Source: CAD feature listing. Evaluate the final solid. Frame: model axes, mm. Face numbers are marked on the shaded views. A direction names the side the tool comes from. Coordinates: 2 decimals unless noted, no trailing zeros. Write each loop counter-clockwise with the first axis right and the second up, starting at its lowest first coordinate (ties: lowest second). Pieces come first, ordered by that corner, then holes. Notation, with made-up numbers: (51.5, -7) - (89.5, -7) arc R20 ccw to (89.5, 0) - close; hole circle Ø11 at (62, 39). An arc over 180 degrees is marked (long way). One line per item, written item: value.
from build123d import *

# Parameters (mm, degrees)
CROQUIS1_R              = 7.55
CROQUIS1_R_2            = 5
SALIENTE_EXTRUIR1_DEPTH = 7
SALIENTE_EXTRUIR2_DEPTH = 51
CROQUIS3_R              = 7.55
SALIENTE_EXTRUIR3_DEPTH = 51
CORTAR_EXTRUIR2_DEPTH   = 14.5
CROQUIS7_R              = 4.1
CORTAR_EXTRUIR3_DEPTH   = 35
CROQUIS8_W              = 8.6
CROQUIS8_H              = 23
CORTAR_EXTRUIR4_DEPTH   = 84
CROQUIS10_R             = 1.55
CORTAR_EXTRUIR7_DEPTH   = 14.5
CORTAR_EXTRUIR8_DEPTH   = 14.5
CROQUIS12_W             = 14.417096231
CROQUIS12_H             = 5
CORTAR_EXTRUIR9_DEPTH   = 14.5
CROQUIS13_W             = 9.25
CROQUIS13_H             = 13.5
SALIENTE_EXTRUIR4_DEPTH = 2.5
REDONDEO2_R             = 2
CROQUIS14_R             = 1
CORTAR_EXTRUIR10_DEPTH  = 4
CROQUIS15_R             = 1.6
CORTAR_EXTRUIR11_DEPTH  = 61.5


with BuildPart() as part:
    # Croquis1 → Saliente-Extruir1 (new body)
    with BuildSketch(Plane(origin=(0, 0, 0), x_dir=(1, 0, 0), z_dir=(0, 1, 0))):
        with BuildLine():
            Line((-11, 0), (-11, 12.5))
            Line((-11, 12.5), (-53.5, 12.5))
            Line((-53.5, 12.5), (-53.5, 26))
            Line((-53.5, 26), (29.5, 26))
            Line((29.5, 26), (29.5, 8))
            Line((29.5, 8), (29.5, 0))
            ThreePointArc((29.5, 0), (21.303512587, -11.735833137), (7.463235294, -8.0808489))
            ThreePointArc((7.463235294, -8.0808489), (-4.410465495, -10.077092543), (-11, 0))
        make_face()
        Circle(CROQUIS1_R, mode=Mode.SUBTRACT)
        with Locations((17, 0)):
            Circle(CROQUIS1_R_2, mode=Mode.SUBTRACT)
    extrude(amount=SALIENTE_EXTRUIR1_DEPTH)

    # Croquis2 → Saliente-Extruir2 (add)
    with BuildSketch(Plane.XZ):
        Polygon((29.5, -26), (29.5, -12.5), (-11, -12.5), (-53.5, -12.5), (-53.5, -26), align=None)
    extrude(amount=SALIENTE_EXTRUIR2_DEPTH)

    # Croquis3 → Saliente-Extruir3 (add)
    with BuildSketch(Plane.XZ):
        with BuildLine():
            Line((-11, 0), (-11, -12.5))
            Line((-11, -12.5), (11, -12.5))
            Line((11, -12.5), (11, 0))
            ThreePointArc((11, 0), (10.077092543, 4.410465495), (7.463235294, 8.0808489))
            ThreePointArc((7.463235294, 8.0808489), (-4.410465495, 10.077092543), (-11, 0))
        make_face()
        Circle(CROQUIS3_R, mode=Mode.SUBTRACT)
    extrude(amount=SALIENTE_EXTRUIR3_DEPTH)

    # Croquis5 → Cortar-Extruir2 (cut, through all)
    with BuildSketch(Plane.XY.offset(-12.5)):
        Polygon((-53.5, 7), (-48.5, 7), (-53.5, 2), align=None)
    extrude(amount=-CORTAR_EXTRUIR2_DEPTH, mode=Mode.SUBTRACT)

    # Croquis7 → Cortar-Extruir3 (cut)
    with BuildSketch(Plane(origin=(29.5, 0, 0), x_dir=(0, 0, -1), z_dir=(1, 0, 0))):
        with Locations((19.25, -1)):
            Circle(CROQUIS7_R)
        with Locations((19.25, -46)):
            Circle(CROQUIS7_R)
    extrude(amount=-CORTAR_EXTRUIR3_DEPTH, mode=Mode.SUBTRACT)

    # Croquis8 → Cortar-Extruir4 (cut, through all)
    with BuildSketch(Plane(origin=(29.5, 0, 0), x_dir=(0, 0, -1), z_dir=(1, 0, 0))):
        with Locations((19.25, -23.5)):
            Rectangle(CROQUIS8_W, CROQUIS8_H)
    extrude(amount=-CORTAR_EXTRUIR4_DEPTH, mode=Mode.SUBTRACT)

    # Croquis10 → Cortar-Extruir7 (cut, through all)
    with BuildSketch(Plane.XY.offset(-12.5)):
        with Locations((-49.5, -6)):
            Circle(CROQUIS10_R)
        with Locations((-18.5, -6)):
            Circle(CROQUIS10_R)
        with Locations((-18.5, -37)):
            Circle(CROQUIS10_R)
    extrude(amount=-CORTAR_EXTRUIR7_DEPTH, mode=Mode.SUBTRACT)

    # Croquis11 → Cortar-Extruir8 (cut, through all)
    with BuildSketch(Plane.XY.offset(-12.5)):
        Polygon((-53.5, -8.669284564), (-53.5, -51), (-25.417096231, -51), (-25.417096231, -33), (-17.334192463, -19), (-25.417096231, -5), (-41.582903769, -5), (-43.7013662, -8.669284564), align=None)
    extrude(amount=-CORTAR_EXTRUIR8_DEPTH, mode=Mode.SUBTRACT)

    # Croquis12 → Cortar-Extruir9 (cut, through all)
    with BuildSketch(Plane.XY.offset(-12.5)):
        with Locations((-18.208548116, -48.5)):
            Rectangle(CROQUIS12_W, CROQUIS12_H)
    extrude(amount=-CORTAR_EXTRUIR9_DEPTH, mode=Mode.SUBTRACT)

    # Croquis13 → Saliente-Extruir4 (add)
    with BuildSketch(Plane.XZ.offset(51)):
        with Locations((24.875, -19.25)):
            Rectangle(CROQUIS13_W, CROQUIS13_H)
    extrude(amount=SALIENTE_EXTRUIR4_DEPTH)

    # Redondeo2
    redondeo2_edges = [part.edges().sort_by_distance(p)[0] for p in [
        (20.25, -53.5, -19.25),
    ]]
    fillet(redondeo2_edges, radius=REDONDEO2_R)

    # Croquis14 → Cortar-Extruir10 (cut)
    with BuildSketch(Plane.XZ.offset(53.5)):
        with Locations((24.25, -14)):
            Circle(CROQUIS14_R)
        with Locations((24.25, -24)):
            Circle(CROQUIS14_R)
    extrude(amount=-CORTAR_EXTRUIR10_DEPTH, mode=Mode.SUBTRACT)

    # Croquis15 → Cortar-Extruir11 (cut, through all)
    with BuildSketch(Plane(origin=(0, 7, 0), x_dir=(1, 0, 0), z_dir=(0, 1, 0))):
        with Locations((17, 8)):
            Circle(CROQUIS15_R)
        with Locations((17, -8)):
            Circle(CROQUIS15_R)
    extrude(amount=-CORTAR_EXTRUIR11_DEPTH, mode=Mode.SUBTRACT)


solid = part.part
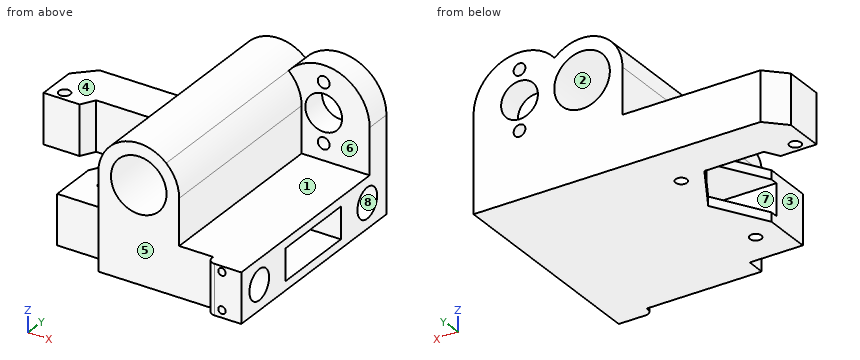
1) Reachability of the marked faces 4, 5, 6, 7 and 8 from +Z, -Z, +X, -X, +Y, -Y: full face, straight path, thin tool, end or side. Return the list, or none.
Values found:
face 4: +Z, -X, +Y, -Y
face 5: +Z, -Z, -X, -Y
face 6: +Z, +X, -Y
face 7: +X, -X
face 8: +X
2) Section query C-C on y = -26. Output: boundary loops of the cut face in (x, z), then the cut area to 3 significant figures.
Values found:
outline: (-21.38, -26) - (29.5, -26) - (29.5, -23.55) - (-21.38, -23.55) - close; (-21.38, -14.95) - (29.5, -14.95) - (29.5, -12.5) - (11, -12.5) - (11, 0) arc R11 ccw to (-11, 0) - (-11, -12.5) - (-21.38, -12.5) - close; hole circle Ø15.1 at (0, 0)
area: 535 mm2
3) Draft query along Z for the marked faces 1, 2 and 3. Return one class per face: released by +Z, released by -Z, zero draft, split by the parting line, or undercut.
Values found:
face 1: released by +Z
face 2: undercut
face 3: zero draft
4) Section query D-D on x = 3. Output: boundary loops of the cut face in (y, z).
Values found:
outline: (-51, -26) - (7, -26) - (7, -6.93) - (-51, -6.93) - close; (-51, 6.93) - (7, 6.93) - (7, 10.58) - (-51, 10.58) - close; hole circle Ø8.2 at (-46, -19.25); hole (-35, -23.55) - (-12, -23.55) - (-12, -14.95) - (-35, -14.95) - close; hole circle Ø8.2 at (-1, -19.25)
5) Section query B-B on x = 17. Output: boundary loops of the cut face in (y, z), then the cut area to 3 significant figures.
Values found:
outline: (-51, -26) - (7, -26) - (7, -9.6) - (0, -9.6) - (0, -12.5) - (-51, -12.5) - close; (0, -6.4) - (7, -6.4) - (7, -5) - (0, -5) - close; (0, 5) - (7, 5) - (7, 6.4) - (0, 6.4) - close; (0, 9.6) - (7, 9.6) - (7, 12.5) - (0, 12.5) - close; hole circle Ø8.2 at (-46, -19.25); hole (-35, -23.55) - (-12, -23.55) - (-12, -14.95) - (-35, -14.95) - close; hole circle Ø8.2 at (-1, -19.25)
area: 540 mm2
6) Section query A-A on z = -19.25. State how many separate pieces and enclosed holes the cut face has, then the cut area to 3 significant figures.
Values found:
separate pieces: 2
enclosed holes: 3
area: 1,630 mm2
7) Material intervals for line 1 (Z direction, x = 24.25, y = -52.15); line 2 (Y direction, x = -18.5, z = -18.75); line 3 (Z direction, x = 23, y = -17), sorted ascending.
Values found:
line 1: -26 to -25, -23 to -15, -13 to -12.5
line 2: -46 to -38.55, -35.45 to -35, -12 to -7.55, -4.45 to 7
line 3: -26 to -23.55, -14.95 to -12.5
8) Contact query for flat-ended pins moving along their axis: P1, Ø10, axis at x = -29.5, y = -39, coming from the -Z side; P2, Ø13, axis at y = -35.5, z = -16.5, coming from the -X side; P3, Ø3.5, axis at x = 17, z = -8, coming from the -Y side; P4, Ø4, axis at y = -47, z = -18, coming from the +X side. Output: stop coordinate, or through.
Values found:
P1: z = -26
P2: x = -25.42
P3: y = 0
P4: x = -5.5
